CAD build for the part. Positions are in the model's coordinates, mm. Give positions to 0.01 mm unless a question says otherwise; leave off trailing zeros. Loops run counter-clockwise (first coordinate to the right, second up) from the corner with the lowest first, then second, coordinate; pieces in that order, holes last.
Item 1: Saw through at A-A on z = -22.5. Give the cut face in (x, y), plus the area to 3 significant figures.
Item 2: Mould opens along X. For faces 1 (the cylindrical face through (-4.336, -19.524, -12.325)), 2 (the flat face through (0, -40, -10)), 3 (the flat face through (-34.803, -19.72, -9.93)) say: released by +X, released by -X, zero draft, split by the parting line, or undercut.
Item 3: Drop flat-ended pins along their axis: P1, Ø6, axis at y = 8.5, z = -4, coming from the +X side; P2, Ø3, axis at y = 8, z = -4, coming from the +X side; P3, Ø6, axis at y = -14, z = -11.5, coming from the -X side. Give the stop position or say it passes through.
Item 4: Probe probe 1 along Y at (x, z) = (0, -13.25); probe 2 along X at (y, z) = (8, -3.25); probe 3 along Y at (x, z) = (-16.5, -11.5). List the from-to ranges inside material, lowest first.
Solid Edge part; units mm, degrees
sketch "Sketch1" plane through (0, 0, 0) normal (0, 0, 1) x (1, 0, 0)
  line L0 (-23.094, -40) -> (23.094, -40)
  line L1 (23.094, -40) -> (46.188, 0)
  line L2 (46.188, 0) -> (23.094, 40)
  line L3 (23.094, 40) -> (-23.094, 40)
  line L4 (-23.094, 40) -> (-46.188, 0)
  line L5 (-46.188, 0) -> (-23.094, -40)
extrude "Protrusion1" add sketch "Sketch1" against normal blind 25
sketch "Sketch2" plane through (0, 0, 0) normal (0, 0, 1) x (1, 0, 0)
  circle A0 centre (0, 0) radius 20
extrude "ExtrudedCutout_1" cut sketch "Sketch2" against normal blind 25
sketch "Sketch3" plane through (0, 0, 0) normal (0, -1, 0) x (1, 0, 0)
  line L0 (46.188, -4.0666) -> (42.3722, 0)
  line L1 (42.3722, 0) -> (46.188, 0)
  line L2 (46.188, 0) -> (46.188, -4.0666)
revolve "RevolvedCutout1" cut sketch "Sketch3" angle 360 about axis through (0, 0, 0) along (0, 0, 1)
sketch "Sketch4" plane through (0, 0, 0) normal (0, -1, 0) x (1, 0, 0)
  line L0 (34.641, -25) -> (46.188, -14.5333)
  line L1 (46.188, -25) -> (46.188, -14.5333)
  line L2 (46.188, -25) -> (34.641, -25)
revolve "RevolvedCutout2" cut sketch "Sketch4" angle 360 about axis through (0, 0, 0) along (0, 0, -1)
Results below:
1. outline: circle Ø74.8 at (0, 0); hole circle Ø40 at (0, 0)
1. area: 3,140 mm2
2. face 1: undercut
2. face 2: zero draft
2. face 3: released by -X
3. P1: stops at x = 43.01
3. P2: stops at x = 42.44
3. P3: stops at x = -39.84
4. probe 1: y = -40 to -20, 20 to 40
4. probe 2: x = -41.57 to -18.33, 18.33 to 41.57
4. probe 3: y = -40 to -11.3, 11.3 to 40
